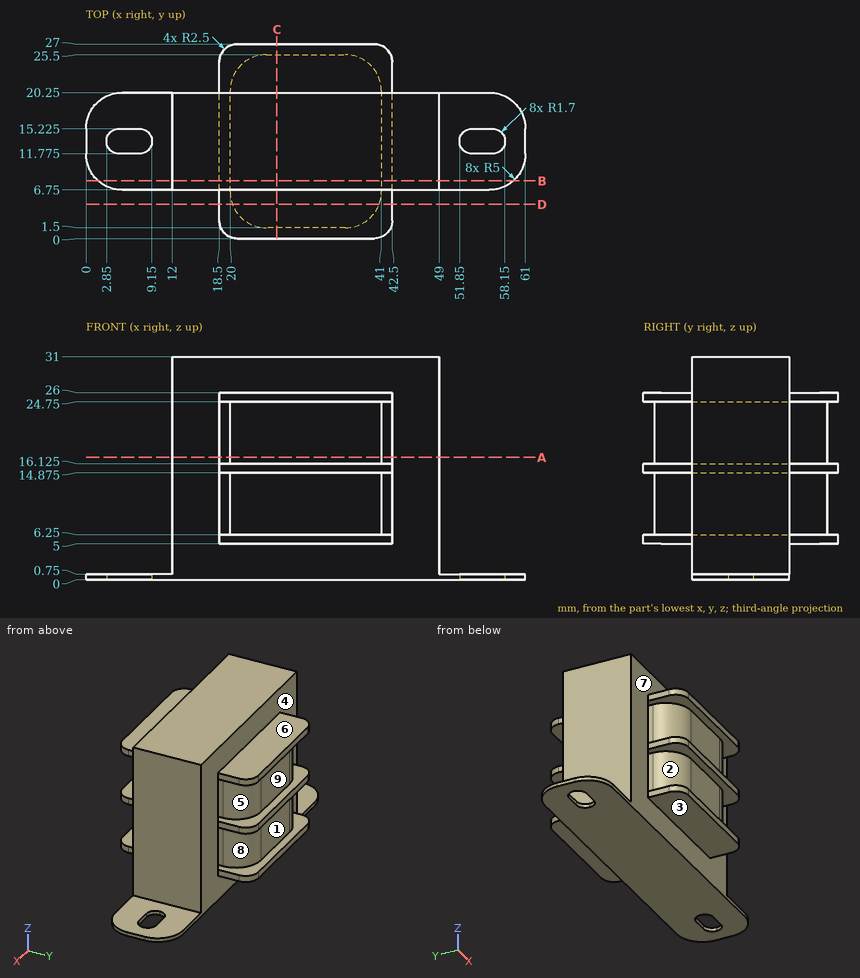
Check sheet for the drawn part. Datum: minimum x, y, z corner. Units: mm. A direction names the side the tool comes from. Coordinates: 2 decimals unless noted, no trailing zeros. Order: outer loops, then holes, each group sorted by start corner. A loop starts at its lowest first (then second) coordinate and runs counter-clockwise, first axis right, second up. Notation, with made-up numbers: (42, 9) - (50, 9) arc R15 ccw to (50, 26) - close; hole circle Ø4 at (-36.75, 86). An arc over 180 degrees is marked (long way). Return JSON: item names as keys, results as strings.
(1) Go/stop test with flat-tipped pins: pin 1 (2 mm diameter, centred on x = 14, z = 8.5, fed in from -Y); pin 2 (4 mm diameter, centred on y = 23.5, z = 22, fed in from -X); pin 3 (8 mm diameter, centred on y = 4, z = 9, fed in from -X). Record where each tip stops, or that it passes through.
Filled sheet:
{"pin 1": "stops at y = 6.75", "pin 2": "stops at x = 20.1", "pin 3": "stops at x = 12"}
(2) Thickness scan on line 1 along Z through (x, y) = (41, 23) (3 decimals); line 2 along X through (y, z) = (16.5, 18.5); line 3 along X through (y, z) = (17, 5.5). Record the ranges inside material, lowest first.
Filled sheet:
{"line 1": "z = 5 to 6.25, 14.875 to 16.125, 24.75 to 26", "line 2": "x = 12 to 18.5, 20 to 41, 42.5 to 49", "line 3": "x = 12 to 49"}
(3) Section check B-B, the plane y = 8. Record the cut outline in (x, z) (3 decimals).
Filled sheet:
{"outline": "(1.693, 0) - (59.307, 0) - (59.307, 0.75) - (49, 0.75) - (49, 31) - (12, 31) - (12, 0.75) - (1.693, 0.75) - close; hole (18.5, 6.25) - (20, 6.25) - (20, 14.875) - (18.5, 14.875) - close; hole (18.5, 16.125) - (20, 16.125) - (20, 24.75) - (18.5, 24.75) - close; hole (41, 6.25) - (42.5, 6.25) - (42.5, 14.875) - (41, 14.875) - close; hole (41, 16.125) - (42.5, 16.125) - (42.5, 24.75) - (41, 24.75) - close"}
(4) Section check C-C, the plane x = 26.5. Record the cut outline in (y, z) (3 decimals).
Filled sheet:
{"outline": "(0, 5) - (6.75, 5) - (6.75, 0) - (20.25, 0) - (20.25, 5) - (27, 5) - (27, 6.25) - (25.5, 6.25) - (25.5, 14.875) - (27, 14.875) - (27, 16.125) - (25.5, 16.125) - (25.5, 24.75) - (27, 24.75) - (27, 26) - (20.25, 26) - (20.25, 31) - (6.75, 31) - (6.75, 26) - (0, 26) - (0, 24.75) - (1.5, 24.75) - (1.5, 16.125) - (0, 16.125) - (0, 14.875) - (1.5, 14.875) - (1.5, 6.25) - (0, 6.25) - close"}
(5) Section check A-A, the plane z = 17. Record the cut outline in (x, y).
Filled sheet:
{"outline": "(12, 6.75) - (18.5, 6.75) - (18.5, 20.25) - (12, 20.25) - close; (20, 6.5) arc R5 ccw to (25, 1.5) - (36, 1.5) arc R5 ccw to (41, 6.5) - (41, 20.5) arc R5 ccw to (36, 25.5) - (25, 25.5) arc R5 ccw to (20, 20.5) - close; (42.5, 6.75) - (49, 6.75) - (49, 20.25) - (42.5, 20.25) - close"}
(6) Access from +Z, -Z, +X, -X, +Y, -Y to the whole of each face (thin tool, end or side, straight path). Record for the marked faces 1, 2, 3, 4 and 5.
Filled sheet:
{"face 1": "+X, -X, +Y", "face 2": "-X, -Y", "face 3": "-Z, +X, -X, -Y", "face 4": "+Y", "face 5": "+X, +Y"}
(7) Section check D-D, the plane y = 4.75. Record the cut outline in (x, z) (3 decimals), and give its area (3 significant figures).
Filled sheet:
{"outline": "(18.5, 5) - (42.5, 5) - (42.5, 6.25) - (40.684, 6.25) - (40.684, 14.875) - (42.5, 14.875) - (42.5, 16.125) - (40.684, 16.125) - (40.684, 24.75) - (42.5, 24.75) - (42.5, 26) - (18.5, 26) - (18.5, 24.75) - (20.316, 24.75) - (20.316, 16.125) - (18.5, 16.125) - (18.5, 14.875) - (20.316, 14.875) - (20.316, 6.25) - (18.5, 6.25) - close", "area": "441 mm^2"}
(8) Mould release check, pull along Z, two halves, no side actions. Record for the marked faces 6, 7, 8 and 9: pulls with the +Z half, pulls with the -Z half, needs draft (parallel to the pull), parting line crosses it, or undercut.
Filled sheet:
{"face 6": "pulls with the +Z half", "face 7": "needs draft", "face 8": "undercut", "face 9": "undercut"}
